Autodesk Inventor part; units mm, degrees
ref_plane "YZ Plane" through (0, 0, 0) normal (1, 0, 0) x (0, 1, 0)
ref_plane "XZ Plane" through (0, 0, 0) normal (0, 1, 0) x (-1, 0, 0)
ref_plane "XY Plane" through (0, 0, 0) normal (0, 0, 1) x (1, 0, 0)
sketch "Sketch2" plane through (0, 0, 0) normal (0, 0, 1) x (1, 0, 0)
  arc A0 (9.9386, -9.7664) -> (20.0614, -9.7664) centre (15, 0) ccw
  arc A1 (20.9272, -9.2665) -> (25.9886, -0.4999) centre (15, 0) ccw
  arc A2 (25.9886, 0.4999) -> (20.9272, 9.2665) centre (15, 0) ccw
  arc A3 (20.0614, 9.7664) -> (9.9386, 9.7664) centre (15, 0) ccw
  arc A4 (9.0728, 9.2665) -> (4.0114, 0.4999) centre (15, 0) ccw
  arc A5 (4.0114, -0.4999) -> (9.0728, -9.2665) centre (15, 0) ccw
  circle A6 centre (15, 0) radius 2.5
  arc A7 (0, -3) -> (12, -15) centre (12, -3) ccw
  circle A8 centre (15, 0) radius 16.1883
  line L0 (31.1883, 0) -> (-118.8117, 0) construction
  line L1 (-118.8117, 0) -> (-118.8117, 35)
  line L2 (17.2352, 16.0332) -> (-118.8117, 35)
  line L3 (-118.8117, 0) -> (-118.8117, -35)
  line L4 (17.2352, -16.0332) -> (-118.8117, -35)
  line L5 (-118.8117, -20) -> (-122.0117, -20)
  line L6 (-122.0117, -20) -> (-122.0117, -5)
  line L7 (-122.0117, -5) -> (-118.8117, -5)
  line L8 (-118.8117, 20) -> (-122.0117, 20)
  line L9 (-122.0117, 20) -> (-122.0117, 5)
  line L10 (-122.0117, 5) -> (-118.8117, 5)
  line L11 (-118.8117, 0) -> (-118.8117, 1.6)
  line L12 (-118.8117, 1.6) -> (-93.8117, 1.6)
  line L13 (-118.8117, 0) -> (-118.8117, -1.6)
  line L14 (-118.8117, -1.6) -> (-93.8117, -1.6)
  line L15 (-93.8117, -1.6) -> (-93.8117, 1.6)
  point P0 (0, 0)
  point P1 (5.2336, -12.9104)
  point P2 (2.0896, -9.7664)
  point P3 (-118.8117, 5)
  point P4 (-118.8117, 20)
extrude "Extrusion1" add sketch "Sketch2" along normal blind 6.2
sketch "Sketch4" plane through (0, 0, 0) normal (0, 0, -1) x (-1, 0, 0)
  line L0 (93.8117, -1.6) -> (93.8117, 1.6)
  line L1 (118.8117, 1.6) -> (93.8117, 1.6)
  line L2 (118.8117, -1.6) -> (93.8117, -1.6)
  line L3 (118.8117, 5) -> (118.8117, -5)
  line L4 (118.8117, 0) -> (118.8117, -35)
  point P0 (0, 0)
extrude "Extrusion2" cut sketch "Sketch4" against normal blind 10
sketch "Sketch5" plane through (0, 0, 0) normal (0, 0, -1) x (-1, 0, 0)
  line L0 (118.8117, -111.6) -> (118.8117, 288.4)
  line L1 (118.8117, -20) -> (118.8117, -35)
  line L2 (118.8117, -24) -> (112.7117, -24)
  line L3 (112.7117, -24) -> (112.7117, -28)
  line L4 (112.7117, -28) -> (118.8117, -28)
  line L5 (118.8117, -28) -> (118.8117, -24)
  line L6 (112.7117, -26) -> (112.7117, -22.5)
  line L7 (112.7117, -22.5) -> (109.5117, -22.5)
  line L8 (112.7117, -26) -> (114.7394, -26) construction
  line L9 (112.7117, -26) -> (112.7117, -29.5)
  line L10 (112.7117, -29.5) -> (109.5117, -29.5)
  line L11 (109.5117, -29.5) -> (109.5117, -22.5)
  line L12 (93.8117, -1.6) -> (93.8117, 1.6)
  line L13 (93.8117, 0) -> (109.9488, 0) construction
  line L14 (118.8117, 111.6) -> (118.8117, -288.4)
  line L15 (118.8117, 20) -> (118.8117, 35)
  line L16 (118.8117, 24) -> (112.7117, 24)
  line L17 (112.7117, 28) -> (118.8117, 28)
  line L18 (112.7117, 26) -> (112.7117, 22.5)
  line L19 (112.7117, 22.5) -> (109.5117, 22.5)
  line L20 (112.7117, 26) -> (112.7117, 29.5)
  line L21 (112.7117, 29.5) -> (109.5117, 29.5)
  line L22 (109.5117, 29.5) -> (109.5117, 22.5)
  point P0 (0, 0)
  point P1 (112.7117, 24)
  point P2 (112.7117, -24)
  dimension "d14" = 6.1
  dimension "d15" = 4
  dimension "d16" = 7
  dimension "d17" = 3.5
  dimension "d18" = 3.2
extrude "Extrusion3" cut sketch "Sketch5" against normal blind 6.2
properties part number "Base"
Design review of the part built by this model. Coordinates are the model's own, in mm. A direction names the side the tool comes from. Give positions to 0.01 mm unless a question says otherwise; leave off trailing zeros. Write each loop counter-clockwise with the first axis right and the second up, starting at its lowest first coordinate (ties: lowest second). Pieces come first, ordered by that corner, then holes.
(1) Tool access review of faces 1 (the face through (-109.512, 26, 3)), 2 (the face through (-120, 5, 3)), 3 (the face through (-118.812, 22, 3)): name each direction out of +Z, -Z, +X, -X, +Y, -Y from which nothing blocks a thin tool from reaching the whole face with its end or side.
Checked values:
face 1: +Z, -Z
face 2: +Z, -Z, -X
face 3: +Z, -Z, -X, +Y
(2) Clearance check with flat-ended pins moving along their axes: pin 1 Ø2.5 at (y, z) = (3.5, 3) entering from -X; pin 2 Ø1.6 at (x, z) = (-121, 2.5) entering from +Y; pin 3 Ø1.6 at (x, z) = (-120.5, 3) entering from -Y. State where each tip first meets the part, or that it passes through.
Checked values:
pin 1: stops at x = -118.81
pin 2: stops at y = 20
pin 3: stops at y = -20
(3) Wall thickness on line 1 along Y through (x, z) = (-114.5, 1.5); line 2 along Y through (x, z) = (-114, 3.5); line 3 along Y through (x, z) = (15, 2.25): over which ranges is each line inside the solid? List them lowest first.
Checked values:
line 1: y = -34.4 to -28, -24 to -1.6, 1.6 to 24, 28 to 34.4
line 2: y = -34.33 to -28, -24 to -1.6, 1.6 to 24, 28 to 34.33
line 3: y = -16.34 to -2.5, 2.5 to 16.34
(4) Add section A-A (y = 0). Give the boundary of the cut face in (x, z), and give its area (3 significant figures).
Checked values:
outline: (-93.81, 0) - (12.5, 0) - (12.5, 6.2) - (-93.81, 6.2) - close; (17.5, 0) - (31.19, 0) - (31.19, 6.2) - (17.5, 6.2) - close
area: 744 mm2
(5) Mouldability with a two-part tool opening along Y and no side actions: class faces 4 (the face through (-120, -20, 3)), 5 (the face through (-120, -5, 3)), 6 (the face through (-122.012, -13, 3)), 7 (the face through (-111, -22.5, 3)) as +Y half, -Y half, draft (parallel to the pull), parting line (faces both ways), or undercut.
Checked values:
face 4: -Y half
face 5: undercut
face 6: draft
face 7: undercut
(6) Add section C-C (x = 15). Give the boundary of the cut face in (y, z).
Checked values:
outline: (-16.34, 0) - (-2.5, 0) - (-2.5, 6.2) - (-16.34, 6.2) - close; (2.5, 0) - (16.34, 0) - (16.34, 6.2) - (2.5, 6.2) - close
(7) Add section D-D (x = -71.5). Give the boundary of the cut face in (y, z), and give its area (3 significant figures).
Checked values:
outline: (-28.4, 0) - (28.4, 0) - (28.4, 6.2) - (-28.4, 6.2) - close
area: 352 mm2
